Work out the finished part from the listing and answer in its coordinate system (mm). A direction names the side the tool comes from. Coordinates: 2 decimals unless noted, no trailing zeros. Loops run counter-clockwise (first coordinate to the right, second up) from the corner with the lowest first, then second, coordinate; pieces in that order, holes last. Notation, with made-up numbers: (-22.75, 17.25) - (15.25, 17.25) arc R19 cw to (15.25, 39.25) - close; hole circle Ø11 at (-39.75, -40). An arc over 180 degrees is marked (long way). Write each question's results on one line, items separated by ' | '. Start each with the question number.
Item 1: A tool of negligible diameter and unlimited length cuts with its end or side. For faces 4 (the face through (8.581, -14.417, 0.76)), 5 (the face through (57.55, 12.99, 0.76)), 6 (the face through (12, -10, 1.5)), 7 (the face through (-31.51, -32.79, 0.76)), from which of +Z, -Z, +X, -X, +Y, -Y can it reach the whole face along a straight path? Write none if from no direction.
Item 2: Consider probe 1 along X at (y, z) = (4.5, 0.4); probe 2 along Y at (x, z) = (21, 1.2); probe 3 along X at (y, z) = (-15, 0.35). Determine where each line is inside the solid, lowest interval first. Write a range as [from, to].
Item 3: Section A-A, the plane x = 22 is taken. Write down the section's boundary in (y, z).
Item 4: For a pull along Y with two mould halves and no side action, classify faces 1 (the face through (57.405, 17.016, 0.76)), 2 (the face through (-31.423, -36.812, 0.76)), 3 (the face through (-16.49, -5.49, 0.76)) as +Y half, -Y half, draft (parallel to the pull), parting line (faces both ways), or undercut.
Item 5: Section C-C, the plane z = 0.85 is taken. Count the separate pieces of the cut face and the enclosed holes in it, plus the area to 3 significant figures.
Item 6: Each of these flat-tipped pins is pushed along its axis until it touches: pin 1 Ø0.8 at (y, z) = (-1, 1) entering from +X; pin 2 Ø0.8 at (y, z) = (2, 0.5) entering from -X. Where does it stop, or does it pass through?
Item 7: Section B-B, the plane y = -24 is taken. Write down the section's boundary in (x, z), plus the area to 3 significant figures.
from build123d import *

# Parameters (mm, degrees)
F0_W     = 28
F0_H     = 18.089384
F1_DEPTH = 1.5
F2_R     = 5
F3_R     = 2


with BuildPart() as f1:
    # F0 (on Top) → F1 (new body)
    with BuildSketch(Plane.XY):
        Polygon((58.006592, 17.586541), (-31.993408, 17.586541), (-31.993408, 12.586541), (-23.993408, 11.175925), (-23.993408, -9.913459), (-23.993408, -31.002843), (-31.993408, -32.413459), (-31.993408, -37.413459), (58.006592, -37.413459), (58.006592, -32.413459), (50.006592, -31.002843), (50.006592, -9.913459), (50.006592, 11.175925), (58.006592, 12.586541), align=None)
        with Locations((-3.993408, -21.958151)):
            Rectangle(F0_W, F0_H, mode=Mode.SUBTRACT)
        with Locations((30.006592, -21.958151)):
            Rectangle(F0_W, F0_H, mode=Mode.SUBTRACT)
        with Locations((-3.993408, 2.131233)):
            Rectangle(F0_W, F0_H, mode=Mode.SUBTRACT)
        with Locations((30.006592, 2.131233)):
            Rectangle(F0_W, F0_H, mode=Mode.SUBTRACT)
    extrude(amount=F1_DEPTH)

    # F2
    f2_edges = [f1.edges().sort_by_distance(p)[0] for p in [
        (44.006592, 11.175925, 0.75),
        (10.006592, 11.175925, 0.75),
        (44.006592, -12.913459, 0.75),
        (10.006592, -12.913459, 0.75),
        (16.006592, 11.175925, 0.75),
        (-17.993408, 11.175925, 0.75),
        (-17.993408, -12.913459, 0.75),
        (16.006592, -12.913459, 0.75),
        (16.006592, -6.913459, 0.75),
        (-17.993408, -6.913459, 0.75),
        (-17.993408, -31.002843, 0.75),
        (16.006592, -31.002843, 0.75),
        (44.006592, -6.913459, 0.75),
        (10.006592, -6.913459, 0.75),
        (44.006592, -31.002843, 0.75),
        (10.006592, -31.002843, 0.75),
    ]]
    fillet(f2_edges, radius=F2_R)

    # F3
    f3_edges = [f1.edges().sort_by_distance(p)[0] for p in [
        (-31.993408, 12.586541, 0.75),
        (-31.993408, -32.413459, 0.75),
        (58.006592, 12.586541, 0.75),
        (58.006592, -32.413459, 0.75),
        (58.006592, 17.586541, 0.75),
        (58.006592, -37.413459, 0.75),
        (-31.993408, -37.413459, 0.75),
        (-31.993408, 17.586541, 0.75),
    ]]
    fillet(f3_edges, radius=F3_R)


solid = f1.part
Answer key:
1) face 4: +Z, -Z | face 5: +Z, -Z, +X | face 6: +Z, +X, -X, +Y, -Y | face 7: +Z, -Z, -X
2) probe 1: x = [-23.99, -17.99], [10.01, 16.01], [44.01, 50.01] | probe 2: y = [-37.41, -31], [-12.91, -6.91], [11.18, 17.59] | probe 3: x = [-23.99, -17.06], [9.07, 16.94], [43.07, 50.01]
3) outline: (-37.41, 0) - (-31, 0) - (-31, 1.5) - (-37.41, 1.5) - close; (-12.91, 0) - (-6.91, 0) - (-6.91, 1.5) - (-12.91, 1.5) - close; (11.18, 0) - (17.59, 0) - (17.59, 1.5) - (11.18, 1.5) - close
4) face 1: +Y half | face 2: -Y half | face 3: undercut
5) separate pieces: 1 | enclosed holes: 4 | area: 2,310 mm^2
6) pin 1: stops at x = 50.01 | pin 2: stops at x = -23.99
7) outline: (-23.99, 0) - (-17.99, 0) - (-17.99, 1.5) - (-23.99, 1.5) - close; (10.01, 0) - (16.01, 0) - (16.01, 1.5) - (10.01, 1.5) - close; (44.01, 0) - (50.01, 0) - (50.01, 1.5) - (44.01, 1.5) - close | area: 27.0 mm^2
